Here's how the part is built. I have some questions about the finished solid (model axes, mm). Give positions to 0.01 mm unless a question says otherwise; leave off trailing zeros. Write each loop counter-clockwise with the first axis right and the second up, starting at its lowest first coordinate (ties: lowest second). Pieces come first, ordered by that corner, then holes. Notation, with made-up numbers: (78.25, 23.5) -> (136.25, 23.5) arc R34 ccw to (136.25, 55.5) -> close; hole circle Ø11 at (-25.5, 41). An arc over 180 degrees is marked (long way). Put each result on its own line as item: value. Start each with the question number.
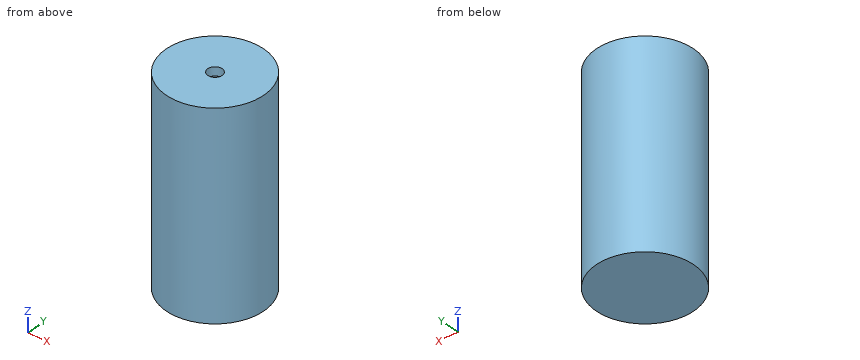
from build123d import *


# Not quite as in the source:
# - a feature names something its author has since deleted; it is built from what else it names


with BuildPart() as f1:
    # F0 (on Front) → F1 (revolve)
    with BuildSketch(Plane.XZ):
        with BuildLine():
            Line((-15, 25.5), (-13, 25.5))
            Line((-13, 25.5), (-2.5, 25.5))
            Line((-2.5, 25.5), (-2.5, 28.5))
            Line((-2.5, 28.5), (-17, 28.5))
            Line((-17, 28.5), (-17, -41.5))
            Line((-17, -41.5), (0, -41.5))
            Line((0, -41.5), (0, -38.5))
            ThreePointArc((0, -38.5), (-9.1923881554, -34.6923881554), (-13, -25.5))
            Line((-13, -25.5), (-13, 22.5))
            Line((-13, 22.5), (-15, 22.5))
            Line((-15, 22.5), (-15, 25.5))
        make_face()
    revolve(axis=Axis((0, 0, -33.5), (0, 0, 1)))


solid = f1.part
1) I want a section at C-C, the plane x = 0. Write out the boundary of the cut face in (y, z).
2) I need wall thicknesses on probe 1 along Y at (x, z) = (0, 24.3); probe 2 along Z at (x, y) = (11, -8); probe 3 along Y at (x, z) = (0, 0). Which ranges of each line are inside material? Lowest first, please.
3) I want a section at A-A, the plane x = -4.5. Write out the boundary of the cut face in (y, z), and give its area (3 significant figures).
4) I want a section at B-B, the plane y = 11. Write out the boundary of the cut face in (x, z).
5) I'm going to push a flat-ended pin straight in: pin 1 Ø2 at (x, z) = (-7.5, -23) entering from -Y. Where does the tip first touch, or does it pass through?
Established:
1. outline: (-17, -41.5) -> (17, -41.5) -> (17, 28.5) -> (2.5, 28.5) -> (2.5, 25.5) -> (15, 25.5) -> (15, 22.5) -> (13, 22.5) -> (13, -25.5) arc R13 cw to (-13, -25.5) -> (-13, 22.5) -> (-15, 22.5) -> (-15, 25.5) -> (-2.5, 25.5) -> (-2.5, 28.5) -> (-17, 28.5) -> close
2. probe 1: y = -17 to -15, 15 to 17
2. probe 2: z = -41.5 to 22.5, 25.5 to 28.5
2. probe 3: y = -17 to -13, 13 to 17
3. outline: (-16.39, -41.5) -> (16.39, -41.5) -> (16.39, 28.5) -> (-16.39, 28.5) -> close; hole (-14.31, 22.5) -> (-12.2, 22.5) -> (-12.2, -25.5) arc R12.2 ccw to (12.2, -25.5) -> (12.2, 22.5) -> (14.31, 22.5) -> (14.31, 25.5) -> (-14.31, 25.5) -> close
3. area: 805 mm2
4. outline: (-12.96, -41.5) -> (12.96, -41.5) -> (12.96, 28.5) -> (-12.96, 28.5) -> close; hole (-10.2, 22.5) -> (-6.93, 22.5) -> (-6.93, -25.5) arc R6.93 ccw to (6.93, -25.5) -> (6.93, 22.5) -> (10.2, 22.5) -> (10.2, 25.5) -> (-10.2, 25.5) -> close
5. pin 1: stops at y = -15.71
